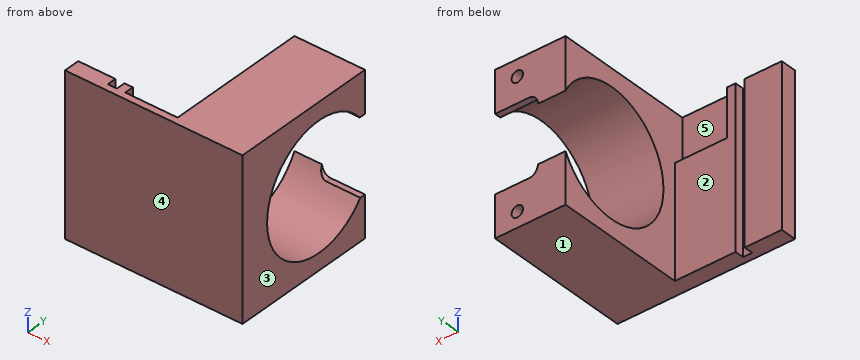
Autodesk Inventor part; units mm, degrees
ref_plane "YZ Plane" through (0, 0, 0) normal (1, 0, 0) x (0, 1, 0)
ref_plane "XZ Plane" through (0, 0, 0) normal (0, 1, 0) x (-1, 0, 0)
ref_plane "XY Plane" through (0, 0, 0) normal (0, 0, 1) x (1, 0, 0)
sketch "Sketch1" plane through (0, 0, 0) normal (0, 1, 0) x (-1, 0, 0)
  line L0 (16.2222, 35.2121) -> (-14.7778, 35.2121)
  line L1 (-14.7778, 35.2121) -> (-14.7778, -34.7879)
  line L2 (-14.7778, -34.7879) -> (16.2222, -34.7879)
  line L3 (16.2222, -34.7879) -> (16.2222, 35.2121)
  point P0 (0, 0)
  dimension "d0" = 70
  dimension "d1" = 31
extrude "Extrusion1" add sketch "Sketch1" along normal blind 60
sketch "Sketch3" plane through (14.7778, 0, 35.2121) normal (1, 0, 0) x (0, 0, -1)
  circle A0 centre (35.2121, 35.5368) radius 27.5
  point P0 (35.2121, 0)
  dimension "d5" = 55
hole "Hole1" at (14.7778, 35.5368, 0) direction (-1, 0, 0) diameter 55 end through all
sketch "Sketch6" plane through (0, 60, 0) normal (0, 1, 0) x (1, 0, 0)
  line L0 (-0.0667, -13.4045) -> (-0.0667, 12.7365)
  line L1 (-16.2222, 0) -> (14.7778, 0) construction
  circle A0 centre (-0.0667, -12.8895) radius 4
  circle A1 centre (-0.0667, 12.5336) radius 4
  point P0 (0, 0)
  point P1 (14.7778, -12.562)
  point P2 (-16.2222, -12.562)
  point P3 (-16.2222, 12.562)
  point P4 (14.7778, 12.562)
  dimension "d42" = 8
  dimension "d43" = 8
sketch "Sketch8" plane through (0, 60, 0) normal (0, 1, 0) x (1, 0, 0)
  line L0 (14.7778, 34.7879) -> (-16.2222, 34.7879) construction
  line L1 (-16.2222, 0) -> (14.7778, 0) construction
  circle A0 centre (5, -28) radius 2
  circle A1 centre (5, 28) radius 2
  point P0 (0, 0)
  dimension "d33" = 4
extrude "Extrusion4" cut sketch "Sketch6" against normal blind 4
sketch "Sketch15" plane through (0, 60, 0) normal (0, 1, 0) x (1, 0, 0)
  arc A0 (-4.0532, -12.562) -> (3.9199, -12.562) centre (-0.0667, -12.8895) ccw
  line L0 (-0.0667, -16.8895) -> (14.7778, -16.8895)
  line L1 (14.7778, 27.5) -> (14.7778, -27.5)
  line L2 (14.7778, -12.562) -> (14.7778, -16.8895)
  line L3 (14.7778, -12.562) -> (3.9199, -12.562)
  line L4 (-0.0667, -12.8895) -> (-0.0667, -12.8895)
  arc A1 (3.9332, 12.562) -> (-4.0666, 12.562) centre (-0.0667, 12.5336) ccw
  line L5 (-0.0667, 16.5336) -> (-0.0667, 12.5336)
  line L6 (3.9332, 12.562) -> (14.7778, 12.562)
  line L7 (14.7778, 12.562) -> (14.7778, 16.5336)
  line L8 (14.7778, 16.5336) -> (-0.0667, 16.5336)
  line L9 (-0.0667, -12.562) -> (14.7778, -12.562)
  line L10 (-0.0667, -12.562) -> (-0.0667, -16.8895)
  line L11 (14.7778, 12.562) -> (-0.0667, 12.5336)
  point P0 (0, 0)
extrude "Extrusion5" cut sketch "Sketch15" against normal blind 4 contours A0 L3 L1 L0 | L1 L6 A1 L8
hole "Hole5" at (5, 60, 28) at (5, 60, -28) direction (0, -1, 0) diameter 5 depth 14
sketch "Sketch18" plane through (0, 0, 0) normal (0, -1, 0) x (1, 0, 0)
  line L0 (-16.2222, -34.7879) -> (-63.2222, -34.7879)
  line L1 (-16.2222, 35.2121) -> (-63.2222, 35.2121)
  line L2 (-63.2222, 35.2121) -> (-63.2222, -34.7879)
  line L3 (-16.2222, -34.7879) -> (-16.2222, 35.2121)
  line L4 (-63.2222, -34.7879) -> (-63.2222, 35.2121)
  point P0 (0, 0)
  dimension "d57" = 47
extrude "Extrusion9" add sketch "Sketch18" against normal blind 2
sketch "Sketch25" plane through (0, 0, 0) normal (0, -1, 0) x (1, 0, 0)
  line L0 (-63.2222, 35.2121) -> (14.7778, 35.2121)
  line L1 (14.7778, 35.2121) -> (14.7778, -34.7879)
  line L2 (14.7778, -34.7879) -> (-63.2222, -34.7879)
  line L3 (-63.2222, -34.7879) -> (-63.2222, 35.2121)
  point P0 (0, 0)
extrude "Extrusion11" add sketch "Sketch25" along normal blind 5
sketch "Sketch29" plane through (0, 2, 0) normal (0, 1, 0) x (1, 0, 0)
  point P0 (0, 0)
sketch "Sketch35" plane through (-63.2222, -5, 35.2121) normal (0, 0, 1) x (1, 0, 0)
  line L0 (42.5, 127.0601) -> (62.5, 127.0601)
  line L1 (62.5, 127.0601) -> (62.5, 71.1035)
  line L2 (62.5, 119.9853) -> (62.5, 78.9853)
  line L3 (62.5, 71.1035) -> (42.5, 71.1035)
  line L4 (42.5, 71.1035) -> (42.5, 127.0601)
  line L5 (42.5, 78.9853) -> (42.5, 119.9853)
  point P0 (63.2222, 5)
extrude "Extrusion20" cut sketch "Sketch35" against normal blind 21
sketch "Sketch37" plane through (0, 2, 0) normal (0, 1, 0) x (1, 0, 0)
  line L0 (-63.2222, -35.2121) -> (-16.2222, -35.2121)
  line L1 (-42.9178, -35.2121) -> (-46.9178, -35.2121)
  line L2 (-46.9178, -35.2121) -> (-46.9178, 34.7879)
  line L3 (-63.2222, 34.7879) -> (14.7778, 34.7879)
  line L4 (-46.9178, 34.7879) -> (-42.9178, 34.7879)
  line L5 (-42.9178, -35.2121) -> (-42.9178, 34.7879)
  point P0 (0, 0)
  dimension "d140" = 4
sketch "Sketch39" plane through (0, 2, 0) normal (0, 1, 0) x (1, 0, 0)
  line L0 (-16.2222, -35.2121) -> (-39.2222, -35.2121)
  line L1 (-39.2222, -35.2121) -> (-39.2222, -14.2121)
  line L2 (-39.2222, -14.2121) -> (-16.2222, -14.2121)
  line L3 (-16.2222, -14.2121) -> (-16.2222, -35.2121)
  point P0 (0, 0)
  dimension "d120" = 23
  dimension "d121" = 21
extrude "Extrusion25" cut sketch "Sketch39" against normal blind 4
extrude "Extrusion26" cut sketch "Sketch37" against normal blind 4
properties part number "Noke_holder_latch"
Verification items for the finished model (mm, model axes). Face numbers are marked on the shaded views. A direction names the side the tool comes from. Round coordinates to 2 decimals unless told otherwise and drop trailing zeros. Write each loop counter-clockwise with the first axis right and the second up, starting at its lowest first coordinate (ties: lowest second). Pieces come first, ordered by that corner, then holes.
(1) Mould release check, pull along X, two halves, no side actions. Record for the marked faces 3, 4 and 5: pulls with the +X half, pulls with the -X half, needs draft (parallel to the pull), parting line crosses it, or undercut.
Returned:
face 3: pulls with the +X half
face 4: needs draft
face 5: undercut
(2) Depth check by flat-ended pin: pin 1 Ø3 at (x, z) = (5, -28) entering from +Y; pin 2 Ø2.5 at (x, z) = (6, -27) entering from +Y; pin 3 Ø10 at (x, z) = (-36.5, -16.5) entering from +Y; pin 4 Ø6.5 at (x, z) = (-31.5, 24.5) entering from +Y. Enter the tip coordinate at first touch or a pass-through.
Returned:
pin 1: stops at y = 46
pin 2: stops at y = 60
pin 3: stops at y = 2
pin 4: stops at y = -2
(3) Section check A-A (y = 50). Enter the section's corners in (x, z), plus the area to 3 significant figures.
Returned:
outline: (-16.22, -34.79) - (14.78, -34.79) - (14.78, -23.39) - (-16.22, -23.39) - close; (-16.22, 23.39) - (14.78, 23.39) - (14.78, 35.21) - (-16.22, 35.21) - close; hole circle Ø5 at (5, -28); hole circle Ø5 at (5, 28)
area: 681 mm2
(4) Material ranges on line 1 (X direction, y = 50.5, z = 28); line 2 (Z direction, x = 5, y = 50.5); line 3 (Z direction, x = 5, y = 52.25), recorded low to high.
Returned:
line 1: x = -16.22 to 2.5, 7.5 to 14.78
line 2: z = -34.79 to -30.5, -25.5 to -23.07, 23.07 to 25.5, 30.5 to 35.21
line 3: z = -34.79 to -30.5, -25.5 to -21.84, 21.84 to 25.5, 30.5 to 35.21
(5) Section check C-C (x = 5). Enter the section's corners in (y, z).
Returned:
outline: (-5, -34.79) - (60, -34.79) - (60, -30.5) - (46, -30.5) - (46, -25.5) - (60, -25.5) - (60, -16.53) - (57.51, -16.53) arc R27.5 cw (long way) to (57.24, 16.89) - (60, 16.89) - (60, 25.5) - (46, 25.5) - (46, 30.5) - (60, 30.5) - (60, 35.21) - (-5, 35.21) - close
(6) Section check D-D (y = 25). Enter the section's corners in (x, z), plus the area to 3 significant figures.
Returned:
outline: (-16.22, -34.79) - (14.78, -34.79) - (14.78, -25.4) - (-16.22, -25.4) - close; (-16.22, 25.4) - (14.78, 25.4) - (14.78, 35.21) - (-16.22, 35.21) - close
area: 595 mm2
(7) Access from +Z, -Z, +X, -X, +Y, -Y to the whole of each face (thin tool, end or side, straight path). Record for the marked faces 1 and 2.
Returned:
face 1: -Z, +X, -X, +Y, -Y
face 2: +Z, -Z, -X, +Y
(8) Section check B-B (z = 0). Enter the section's corners in (x, y), plus the area to 3 significant figures.
Returned:
outline: (-63.22, -5) - (14.78, -5) - (14.78, 8.04) - (-16.22, 8.04) - (-16.22, 2) - (-42.92, 2) - (-42.92, -2) - (-46.92, -2) - (-46.92, 2) - (-63.22, 2) - close
area: 717 mm2
